```python
from build123d import *

# Parameters (mm, degrees)
SKETCH1_W           = 24
SKETCH1_H           = 24
SKETCH1_W_2         = 20.5
SKETCH1_H_2         = 20.5
BOSS_EXTRUDE1_DEPTH = 48.5
CUT_EXTRUDE1_START  = -48.5
SKETCH1_4_W         = 20.5
SKETCH1_4_H         = 20.5
CUT_EXTRUDE1_DEPTH  = 40
CHAMFER2_SIZE       = 3


with BuildPart() as part:
    # Sketch1 → Boss-Extrude1 (new, symmetric)
    # profile 1 of 2: a face of its own
    with BuildSketch(Plane(origin=(0, 0, 0), x_dir=(1, 0, 0), z_dir=(0, 1, 0))):
        Rectangle(SKETCH1_W, SKETCH1_H)
        Rectangle(SKETCH1_W_2, SKETCH1_H_2, mode=Mode.SUBTRACT)
    # profile 2 of 2: a face of its own
    with BuildSketch(Plane(origin=(0, 0, 0), x_dir=(1, 0, 0), z_dir=(0, 1, 0))):
        Rectangle(SKETCH1_W_2, SKETCH1_H_2)
    extrude(amount=BOSS_EXTRUDE1_DEPTH, both=True)

    # Sketch1<4> → Cut-Extrude1 (cut)
    with BuildSketch(Plane(origin=(0, 0, 0), x_dir=(1, 0, 0), z_dir=(0, 1, 0)).offset(CUT_EXTRUDE1_START)):
        Rectangle(SKETCH1_4_W, SKETCH1_4_H)
    extrude(amount=CUT_EXTRUDE1_DEPTH, mode=Mode.SUBTRACT)

    # Sketch3 → Cut-Revolve1 (revolve, cut)
    with BuildSketch(Plane.XY):
        with BuildLine():
            Line((-8.947765084, 48.5), (0, 48.5))
            Line((0, 48.5), (0, 43.25))
            ThreePointArc((0, 43.25), (-5.18712348, 44.659397645), (-8.947765084, 48.5))
        make_face()
    revolve(axis=Axis((0, 64.835592649, 0), (0, -1, 0)), mode=Mode.SUBTRACT)

    # Chamfer2
    chamfer2_edges = [part.edges().sort_by_distance(p)[0] for p in [
        (12, 48.5, 0),
        (0, 48.5, -12),
        (-12, 48.5, 0),
        (0, 48.5, 12),
    ]]
    chamfer(chamfer2_edges, length=CHAMFER2_SIZE)


solid = part.part
```
Could you check a few things on this model? Use its own coordinates, in mm. A direction names the side the tool comes from. Give positions to 0.01 mm unless a question says otherwise; leave off trailing zeros. Loops run counter-clockwise (first coordinate to the right, second up) from the corner with the lowest first, then second, coordinate; pieces in that order, holes last. Notation, with made-up numbers: (66.25, 5.25) -> (107.25, 5.25) arc R32 ccw to (107.25, 37.25) -> close; hole circle Ø5 at (58, 62). An arc over 180 degrees is marked (long way). Put each result on its own line as item: value.
(1) Imagine slicing it at A-A on y = -28. Write out the boundary of the cut face in (x, z), plus the area to 3 significant figures.
Computed:
outline: (-12, -12) -> (12, -12) -> (12, 12) -> (-12, 12) -> close; hole (-10.25, -10.25) -> (10.25, -10.25) -> (10.25, 10.25) -> (-10.25, 10.25) -> close
area: 156 mm^2
(2) I'm going to push flat-ended pins straight in: pin 1 Ø10 at (x, z) = (-2, 0) entering from -Y; pin 2 Ø6 at (x, z) = (3, 5) entering from +Y. Where does each tip first touch, or does it pass through?
Computed:
pin 1: y = -8.5
pin 2: y = 48.3
(3) Imagine slicing it at C-C on z = 3.75. Write out the boundary of the cut face in (x, y), plus the area to 3 significant figures.
Computed:
outline: (-12, -48.5) -> (-10.25, -48.5) -> (-10.25, -8.5) -> (10.25, -8.5) -> (10.25, -48.5) -> (12, -48.5) -> (12, 45.5) -> (9, 48.5) -> (8.12, 48.5) arc R9.54 cw to (-8.12, 48.5) -> (-9, 48.5) -> (-12, 45.5) -> close
area: 1,450 mm^2
(4) Please list where these lines run through material, in increasing order: probe 1 along X at (y, z) = (-30.5, 7.5); probe 2 along Y at (x, z) = (8, 6.25). Write a range as [from, to].
Computed:
probe 1: [-12, -10.25], [10.25, 12]
probe 2: [-8.5, 48.5]
(5) Imagine slicing it at B-B on x = 5.5. Write out the boundary of the cut face in (y, z), plus the area to 3 significant figures.
Computed:
outline: (-48.5, -12) -> (45.5, -12) -> (48.5, -9) -> (48.5, -7.06) arc R8.65 cw to (48.5, 7.06) -> (48.5, 9) -> (45.5, 12) -> (-48.5, 12) -> (-48.5, 10.25) -> (-8.5, 10.25) -> (-8.5, -10.25) -> (-48.5, -10.25) -> close
area: 1,460 mm^2
(6) Thinking about a two-plate mould opening in X: for faces 1 (the face through (0, -8.5, 0)), 2 (the face through (10.5, -48.5, -0.2)), 3 (the face through (-12, -1, 0)), which applies, pulls with the +X half, pulls with the -X half, needs draft (parallel to the pull), parting line crosses it, or undercut?
Computed:
face 1: undercut
face 2: needs draft
face 3: pulls with the -X half
(7) For faces 4 (the face through (-7, 48.5, 6)), 5 (the face through (-10.25, -29, 0)), which set-ups out of +Z, -Z, +X, -X, +Y, -Y let a thin tool reach every point of the face, with its end or its side?
Computed:
face 4: +Z, -Z, +X, -X, +Y
face 5: -Y
